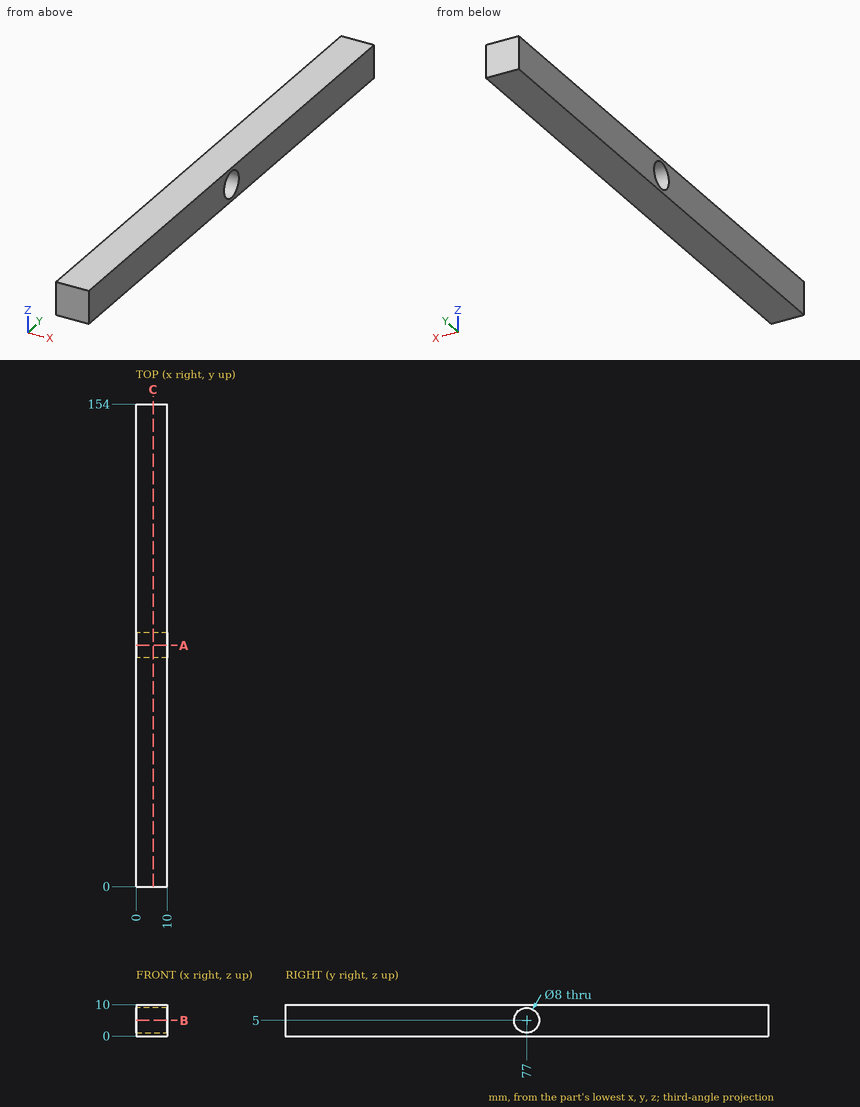
Could you check a few things on this drawing? It's one solid part, dimensions in mm from its lowest x, y, z. Give positions to 0.01 mm unless a question says otherwise; leave off trailing zeros. Write each loop counter-clockwise with the first axis right and the second up, starting at its lowest first coordinate (ties: lowest second). Pieces come first, ordered by that corner, then holes. Notation, with made-up numbers: (2.5, 26) -> (26.5, 26) arc R32 cw to (26.5, 55) -> close; hole circle Ø2 at (31.25, -0.5). An arc over 180 degrees is marked (long way). Answer as a JSON object with one key per item and string values.
Q1. Suppose I cut it at C-C on x = 5.5. Write out the boundary of the cut face in (y, z), then the cut area to 3 significant figures.
Taken from the geometry:
{"outline": "(0, 0) -> (154, 0) -> (154, 10) -> (0, 10) -> close; hole circle Ø8 at (77, 5)", "area": "1,490 mm²"}
Q2. Suppose I cut it at A-A on y = 77. Write out the boundary of the cut face in (x, z), then the cut area to 3 significant figures.
Taken from the geometry:
{"outline": "(0, 0) -> (10, 0) -> (10, 1) -> (0, 1) -> close; (0, 9) -> (10, 9) -> (10, 10) -> (0, 10) -> close", "area": "20.0 mm²"}
Q3. Please list where these lines run through material, in increasing order: L1, parallel to Z at x = 4.75, y = 77; L2, parallel to Y at x = 5, z = 5; L3, parallel to Y at x = 3.75, z = 8.5.
Taken from the geometry:
{"L1": "z = 0 to 1, 9 to 10", "L2": "y = 0 to 73, 81 to 154", "L3": "y = 0 to 75.06, 78.94 to 154"}
Q4. Suppose I cut it at B-B on z = 5. Write out the boundary of the cut face in (x, y), then the cut area to 3 significant figures.
Taken from the geometry:
{"outline": "(0, 0) -> (10, 0) -> (10, 73) -> (0, 73) -> close; (0, 81) -> (10, 81) -> (10, 154) -> (0, 154) -> close", "area": "1,460 mm²"}
Q5. Will these pins go through, and if not, where does the flat tip stop? pin 1 Ø4 at (x, y) = (1.5, 40.5) entering from -Z; pin 2 Ø5 at (y, z) = (77, 5) entering from +X.
Taken from the geometry:
{"pin 1": "stops at z = 0", "pin 2": "passes through"}
